Autodesk Inventor part; units mm, degrees
ref_plane "YZ Plane" through (0, 0, 0) normal (1, 0, 0) x (0, 1, 0)
ref_plane "XZ Plane" through (0, 0, 0) normal (0, 1, 0) x (-1, 0, 0)
ref_plane "XY Plane" through (0, 0, 0) normal (0, 0, 1) x (1, 0, 0)
sketch "Sketch2" plane through (0, 0, 0) normal (0, 0, 1) x (1, 0, 0)
  line L0 (0, 0) -> (0, -18) construction
  line L1 (-9, 0) -> (-9, -18)
  line L2 (9, -18) -> (9, 0)
  arc A0 (9, 0) -> (-9, 0) centre (0, 0) ccw construction
  arc A1 (-9, -18) -> (9, -18) centre (0, -18) ccw
  arc A2 (6.5, -18) -> (-6.5, -18) centre (0, -18) ccw
  circle A3 centre (0, -18) radius 5 construction
  line L3 (-9, 0) -> (9, 0)
  line L4 (9, -18) -> (6.5, -18)
  arc A4 (-6.5, -18) -> (0, -24.5) centre (0, -18) ccw
  arc A5 (0, -24.5) -> (6.5, -18) centre (0, -18) ccw
  line L5 (-6.5, -18) -> (-9, -18)
  line L6 (6.5, -18) -> (-6.5, -18) construction
  line L7 (9, -18) -> (6.5, -18)
  line L8 (-9, -18) -> (-6.5, -18)
  point P0 (0, -9)
  dimension "d2" = 2.5
  dimension "d3" = 10
  dimension "d4" = 1.5
  dimension "d5" = 18
extrude "Extrusion1" add sketch "Sketch2" along normal mid plane 8 contours L3 L2 L4 A2 L5 L1 | L5 A4 A5 L4 A1
sketch "Sketch3" plane through (-9, 0, 4) normal (0, 1, 0) x (1, 0, 0)
  line L0 (-7, 0) -> (25, 0)
  line L1 (25, 0) -> (25, 8)
  line L2 (25, 8) -> (-7, 8)
  line L3 (-7, 8) -> (-7, 0)
  line L4 (-7, 0) -> (25, 8) construction
  line L5 (25, 0) -> (-7, 8) construction
  line L6 (0, 8) -> (18, 8)
  line L7 (0, 8) -> (0, 0)
  point P0 (9, 4)
  dimension "d8" = 7
extrude "Extrusion2" add sketch "Sketch3" against normal blind 2
sketch "Sketch4" plane through (-9, -2, 4) normal (0, -1, 0) x (1, 0, 0)
  line L0 (18, -8) -> (0, -8) construction
  line L1 (-7, 0) -> (0, 0) construction
  line L2 (-7, -8) -> (-7, 0) construction
  line L3 (0, 0) -> (18, 0) construction
  line L4 (25, 0) -> (25, -8) construction
  line L5 (25, -8) -> (18, -8) construction
  line L6 (0, -8) -> (0, 0) construction
  line L7 (0, -8) -> (-7, -8) construction
  line L8 (18, 0) -> (25, 0) construction
  line L9 (18, 0) -> (18, -8) construction
  line L10 (0, 0) -> (0, -8)
  line L11 (0, 0) -> (-7, 0)
  line L12 (-7, 0) -> (-7, -8)
  line L13 (-7, -8) -> (0, -8)
  line L14 (18, -8) -> (18, 0)
  line L15 (18, -8) -> (25, -8)
  line L16 (25, -8) -> (25, 0)
  line L17 (25, 0) -> (18, 0)
  point P0 (-3.5, -4)
  point P1 (21.5, -4)
  point P2 (21.5, 0)
  point P3 (-3.5, 0)
  point P4 (25, -4)
  point P5 (25, -4)
hole "Hole1" at (-12.5, -2, 0) at (12.5, -2, 0) direction (0, 1, 0) diameter 3.4 end through all
chamfer "Chamfer2" distance 1 angle 45 2 edges at (0, -11.5, -4) (0, -11.5, 4)
properties part number "driver gear stopper"
Here's how the part is built. I have some questions about the finished solid (model axes, mm). A direction names the side the tool comes from. Give positions to 0.01 mm unless a question says otherwise; leave off trailing zeros. Loops run counter-clockwise (first coordinate to the right, second up) from the corner with the lowest first, then second, coordinate; pieces in that order, holes last. Notation, with made-up numbers: M 43,-8 L 80,-8 A11 cw 80,-2 Z; hole C 26,-7.5 d4. An arc over 180 degrees is marked long. Put each result on its own line as item: value. Start each with the question number.
(1) I want a section at A-A on x = 0. Please give me the cut outline in (y, z).
(2) For faces 1 (the flat face through (-9, -10, 0)), 2 (the flat face through (0, -7, 4)), 3 (the flat face through (9, -10, 0)), which set-ups out of +Z, -Z, +X, -X, +Y, -Y let a thin tool reach every point of the face, with its end or its side?
(3) Will these pins go through, and if not, where does the flat tip stop? pin 1 Ø3 at (x, z) = (11.5, -2) entering from -Y; pin 2 Ø11.5 at (x, y) = (0, -18) entering from -Z; pin 3 Ø4 at (y, z) = (-7, 0) entering from +X; pin 4 Ø1.5 at (y, z) = (-13.5, -2) entering from -X.
(4) I want a section at B-B on x = 12. Please give me the cut outline in (y, z), then the cut area to 3 significant figures.
(5) I need wall thicknesses on line 1 along X through (y, z) = (-1.25, 0); line 2 along X through (y, z) = (-18, -0.1); line 3 along Y through (x, z) = (0, -1.2). Which ranges of each line are inside material? Lowest first, please. Write a range as [from, to].
(6) If we mould it in two halves opening along Y, with no side actions, what happens to faces 4 (the cylindrical face through (0.286, -11.506, 0.042)), 5 (the cylindrical face through (0, -27, 0)), 6 (the cylindrical face through (-14.186, -0.986, 0.221))? For each: +Y half, -Y half, draft (parallel to the pull), parting line (faces both ways), or undercut.
(7) I want a section at C-C on y = -10. Please give me the cut outline in (x, z), then the cut area to 3 significant figures.
Answer block:
1. outline: M -27,-4 L -25.5,-4 L -24.5,-3 L -24.5,3 L -25.5,4 L -27,4 Z; M -11.5,-3 L -10.5,-4 L 0,-4 L 0,4 L -10.5,4 L -11.5,3 Z
2. face 1: +Z, -Z, -X, -Y
2. face 2: +Z, +X, -X, +Y, -Y
2. face 3: +Z, -Z, +X, -Y
3. pin 1: y = -2
3. pin 2: through
3. pin 3: x = 9
3. pin 4: x = -9
4. outline: M -2,-4 L 0,-4 L 0,-1.62 L -2,-1.62 Z; M -2,1.62 L 0,1.62 L 0,4 L -2,4 Z
4. area: 9.50 mm^2
5. line 1: [-16, -14.2], [-10.8, 10.8], [14.2, 16]
5. line 2: [-9, -6.5], [6.5, 9]
5. line 3: [-27, -24.5], [-11.5, 0]
6. face 4: undercut
6. face 5: -Y half
6. face 6: draft
7. outline: M -9,-4 L 9,-4 L 9,4 L -9,4 Z
7. area: 144 mm^2
